For this review, take the finished solid that the model builds, in its own axes (mm). Face numbers are marked on the shaded views. A direction names the side the tool comes from. Coordinates: 2 decimals unless noted, no trailing zeros. Write each loop counter-clockwise with the first axis right and the second up, starting at its lowest first coordinate (ties: lowest second). Pieces come first, ordered by that corner, then holes. Notation, with made-up numbers: (-6.5, 10) - (6.5, 10) arc R22 cw to (6.5, 23) - close; hole circle Ø3 at (44.25, 77.5). An arc over 180 degrees is marked (long way). Use one line per item in the form item = value. Start each with the question number.
1) For L1, parallel to Y at x = 0, z = 3; L2, parallel to Z at x = 9.5, y = 13; L3, parallel to Y at x = 20.5, z = 1, list the stretches that pass through material, from the lowest coordinate up. Write a range as from..to.
2) We need section D-D (z = 10). Give the boundary of the cut face in (x, y), plus the area to 3 significant figures.
3) We need section B-B (y = -2.5). Give the boundary of the cut face in (x, z), plus the area to 3 significant figures.
4) We need section C-C (x = 16). Give the boundary of the cut face in (y, z), plus the area to 3 significant figures.
5) Insertion check: P1, Ø0.6, axis at y = -24, z = 1.5, coming from the -X side; P2, Ø8, axis at x = -1, y = 17.5, coming from the +Z side; P3, Ø0.6, axis at x = -24.5, z = 1, coming from the +Y side. Each pin has a flat end and moves straight along its axis. Give the tip position at first contact, or say it passes through.
6) We need section A-A (x = -23). Give the boundary of the cut face in (y, z).
7) Tool access review of the marked faces 1 and 2: name each direction out of +Z, -Z, +X, -X, +Y, -Y from which nothing blocks a thin tool from reaching the whole face with its end or side.
```python
from build123d import *

# Parameters (mm, degrees)
SKETCH_R           = 27
SKETCH_R_2         = 3.2
PAD_DEPTH          = 2
SKETCH001_R        = 5.161315
SKETCH001_R_2      = 3.2
PAD001_DEPTH       = 9
POCKET_DEPTH       = 156.312374
POLARPATTERN_COUNT = 8


with BuildPart() as part:
    # Sketch → Pad (new body)
    with BuildSketch(Plane.XY):
        Circle(SKETCH_R)
        Circle(SKETCH_R_2, mode=Mode.SUBTRACT)
    extrude(amount=PAD_DEPTH)

    # Sketch001 (on Face4 of Pad) → Pad001 (join)
    with BuildSketch(Plane.XY.offset(2)):
        with Locations((-8.6e-05, 0.038685)):
            Circle(SKETCH001_R)
        Circle(SKETCH001_R_2, mode=Mode.SUBTRACT)
    extrude(amount=PAD001_DEPTH)

    # Sketch002 (on Face3 of Pad001) → Pocket (cut, through all)
    with BuildSketch(Plane.XY.offset(2)):
        with BuildLine():
            Line((0, 32.043877), (0, 18))
            ThreePointArc((6.888302, 16.629832), (3.511626, 17.654135), (0, 18))
            Line((6.888302, 16.629832), (12.262661, 29.604683))
            Line((0, 32.043877), (12.262661, 29.604683))
        make_face()
    pocket = extrude(amount=-POCKET_DEPTH, mode=Mode.SUBTRACT)

    # PolarPattern: Pocket ×8 about axis
    polarpattern_axis = Axis((0, 0, 2), (0, 0, 1))
    for i in range(1, POLARPATTERN_COUNT):
        add(pocket.rotate(polarpattern_axis, i * 360 / POLARPATTERN_COUNT), mode=Mode.SUBTRACT)


solid = part.part
```
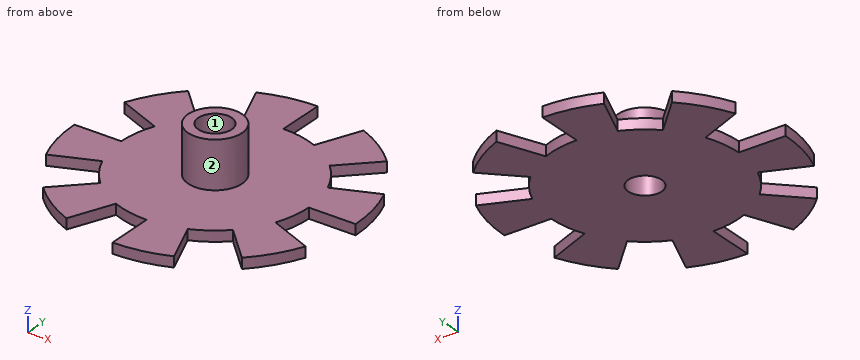
Determined:
q1.L1 = -5.12..-3.2, 3.2..5.2
q1.L2 = 0..2
q1.L3 = -17.57..-8.49, 0..8.49
q2.outline = circle Ø10.32 at (0, 0.04); hole circle Ø6.4 at (0, 0)
q2.area = 51.5 mm²
q3.outline = (-26.88, 0) - (-2, 0) - (-2, 11) - (-4.49, 11) - (-4.49, 2) - (-26.88, 2) - close; (2, 0) - (17.83, 0) - (17.83, 2) - (4.49, 2) - (4.49, 11) - (2, 11) - close
q3.area = 126 mm²
q4.outline = (-16, 0) - (8.25, 0) - (8.25, 2) - (-16, 2) - close; (16, 0) - (21.75, 0) - (21.75, 2) - (16, 2) - close
q4.area = 60.0 mm²
q5.P1 = -12.93
q5.P2 = 2
q5.P3 = 11.97
q6.outline = (-9.53, 0) - (0, 0) - (0, 2) - (-9.53, 2) - close; (9.53, 0) - (14.14, 0) - (14.14, 2) - (9.53, 2) - close
q7.face_1 = +Z, -Z
q7.face_2 = +Z
